```python
from build123d import *

# Parameters (mm, degrees)
SKETCH1_R              = 1.875
SKETCH1_R_2            = 5
BOSS_EXTRUDE1_DEPTH    = 3
CUT_EXTRUDE1_OUTLINE_R = 1.5
CUT_EXTRUDE1_DEPTH     = 3
LPATTERN1_COUNT        = 4
LPATTERN1_PITCH        = 22.666666667
SKETCH1_4_W            = 20
SKETCH1_4_H            = 3
SKETCH1_4_W_2          = 26
BOSS_EXTRUDE2_DEPTH    = 15


# Read off the part's stored shape, not the designer's step: Cut-Extrude1
with BuildPart() as part:
    # Sketch1 → Boss-Extrude1 (new body)
    with BuildSketch(Plane.XY):
        Polygon((77, 130), (63, 130), (63, 127), (37, 127), (37, 130), (23, 130), (23, 127), (3, 127), (3, 130), (0, 130), (0, 0), (100, 0), (100, 130), (97, 130), (97, 127), (77, 127), align=None)
        with Locations((25, 5.75)):
            Circle(SKETCH1_R, mode=Mode.SUBTRACT)
        with Locations((75, 5.75)):
            Circle(SKETCH1_R, mode=Mode.SUBTRACT)
        with BuildLine():
            ThreePointArc((37, 123), (30, 116), (23, 123))
            Line((23, 123), (25, 123))
            ThreePointArc((25, 123), (30, 128), (35, 123))
            Line((35, 123), (37, 123))
        make_face(mode=Mode.SUBTRACT)
        with Locations((70, 123)):
            Circle(SKETCH1_R_2, mode=Mode.SUBTRACT)
    extrude(amount=BOSS_EXTRUDE1_DEPTH)

    # Cut-Extrude1 outline → Cut-Extrude1 (cut)
    with BuildSketch(Plane.XY):
        with Locations((22, 76)):
            Circle(CUT_EXTRUDE1_OUTLINE_R)
        with Locations((10, 92)):
            Circle(CUT_EXTRUDE1_OUTLINE_R)
    cut_extrude1 = extrude(amount=CUT_EXTRUDE1_DEPTH, mode=Mode.SUBTRACT)

    # LPattern1: Cut-Extrude1 ×4
    with Locations(*[(i * LPATTERN1_PITCH, 0, 0) for i in range(1, LPATTERN1_COUNT)]):
        add(cut_extrude1, mode=Mode.SUBTRACT)

    # Sketch1<4> → Boss-Extrude2 (add)
    with BuildSketch(Plane.XY):
        Polygon((0, 130), (0, 90), (3, 90), (3, 127), (3, 130), align=None)
        with Locations((13, 128.5)):
            Rectangle(SKETCH1_4_W, SKETCH1_4_H)
        Polygon((97, 90), (100, 90), (100, 130), (97, 130), (97, 127), align=None)
        with Locations((87, 128.5)):
            Rectangle(SKETCH1_4_W, SKETCH1_4_H)
        with BuildLine():
            Line((77, 127), (77, 130))
            Line((77, 130), (70, 130))
            ThreePointArc((70, 130), (74.949747468, 127.949747468), (77, 123))
            Line((77, 123), (77, 127))
        make_face()
        with BuildLine():
            ThreePointArc((63, 123), (65.050252532, 127.949747468), (70, 130))
            Line((70, 130), (63, 130))
            Line((63, 130), (63, 127))
            Line((63, 127), (63, 123))
        make_face()
        with BuildLine():
            ThreePointArc((77, 123), (74.949747468, 127.949747468), (70, 130))
            ThreePointArc((70, 130), (65.050252532, 127.949747468), (63, 123))
            Line((63, 123), (65, 123))
            ThreePointArc((65, 123), (70, 128), (75, 123))
            Line((75, 123), (77, 123))
        make_face()
        with BuildLine():
            ThreePointArc((63, 123), (70, 116), (77, 123))
            Line((77, 123), (75, 123))
            ThreePointArc((75, 123), (70, 118), (65, 123))
            Line((65, 123), (63, 123))
        make_face()
        with BuildLine():
            ThreePointArc((77, 123), (74.949747468, 127.949747468), (70, 130))
            ThreePointArc((70, 130), (65.050252532, 127.949747468), (63, 123))
            Line((63, 123), (65, 123))
            ThreePointArc((65, 123), (70, 128), (75, 123))
            Line((75, 123), (77, 123))
        make_face()
        with BuildLine():
            ThreePointArc((63, 123), (70, 116), (77, 123))
            Line((77, 123), (75, 123))
            ThreePointArc((75, 123), (70, 118), (65, 123))
            Line((65, 123), (63, 123))
        make_face()
        with Locations((50, 128.5)):
            Rectangle(SKETCH1_4_W_2, SKETCH1_4_H)
        with BuildLine():
            Line((37, 130), (30, 130))
            ThreePointArc((30, 130), (34.949747468, 127.949747468), (37, 123))
            Line((37, 123), (37, 127))
            Line((37, 127), (37, 130))
        make_face()
        with BuildLine():
            Line((30, 130), (23, 130))
            Line((23, 130), (23, 127))
            Line((23, 127), (23, 123))
            ThreePointArc((23, 123), (25.050252532, 127.949747468), (30, 130))
        make_face()
        with BuildLine():
            ThreePointArc((37, 123), (34.949747468, 127.949747468), (30, 130))
            ThreePointArc((30, 130), (25.050252532, 127.949747468), (23, 123))
            Line((23, 123), (25, 123))
            ThreePointArc((25, 123), (30, 128), (35, 123))
            Line((35, 123), (37, 123))
        make_face()
        with BuildLine():
            Line((25, 123), (23, 123))
            ThreePointArc((23, 123), (30, 116), (37, 123))
            Line((37, 123), (35, 123))
            ThreePointArc((35, 123), (30, 118), (25, 123))
        make_face()
        with BuildLine():
            ThreePointArc((37, 123), (34.949747468, 127.949747468), (30, 130))
            ThreePointArc((30, 130), (25.050252532, 127.949747468), (23, 123))
            Line((23, 123), (25, 123))
            ThreePointArc((25, 123), (30, 128), (35, 123))
            Line((35, 123), (37, 123))
        make_face()
        with BuildLine():
            Line((25, 123), (23, 123))
            ThreePointArc((23, 123), (30, 116), (37, 123))
            Line((37, 123), (35, 123))
            ThreePointArc((35, 123), (30, 118), (25, 123))
        make_face()
    extrude(amount=BOSS_EXTRUDE2_DEPTH)


solid = part.part
```
Input: part model. Units: mm. Frame: model coordinates. A direction names the side the tool comes from. Give positions to 0.01 mm unless a question says otherwise; leave off trailing zeros. Order: outer loops, then holes, each group sorted by start corner. A loop starts at its lowest first (then second) coordinate and runs counter-clockwise, first axis right, second up.
1. Section A-A on y = 76. Return the cut outline in (x, z), and give its area (3 significant figures).
Derived:
outline: (0, 0) - (20.5, 0) - (20.5, 3) - (0, 3) - close; (23.5, 0) - (43.17, 0) - (43.17, 3) - (23.5, 3) - close; (46.17, 0) - (65.83, 0) - (65.83, 3) - (46.17, 3) - close; (68.83, 0) - (88.5, 0) - (88.5, 3) - (68.83, 3) - close; (91.5, 0) - (100, 0) - (100, 3) - (91.5, 3) - close
area: 264 mm2
2. Section C-C on z = 9.25. Return the cut outline in (x, y).
Derived:
outline: (0, 90) - (3, 90) - (3, 127) - (23, 127) - (23, 123) arc R7 ccw to (37, 123) - (37, 127) - (63, 127) - (63, 123) arc R7 ccw to (77, 123) - (77, 127) - (97, 127) - (97, 90) - (100, 90) - (100, 130) - (0, 130) - close; hole circle Ø10 at (30, 123); hole circle Ø10 at (70, 123)
3. Pin query (flat end, axial travel): pin 1 (4 mm diameter, centred on x = 22, y = 76, fed in from +Z); pin 2 (2.5 mm diameter, centred on x = 2, z = 10.5, fed in from -Y); pin 3 (1.5 mm diameter, centred on x = 40.5, z = 12, fed in from -Y). Return the tip coordinate at first contact, or that it passes through.
Derived:
pin 1: stops at z = 3
pin 2: stops at y = 90
pin 3: stops at y = 127
4. Section D-D on y = 5.75. Return the cut outline in (x, z) (3 decimals), and give its area (4 significant figures).
Derived:
outline: (0, 0) - (23.125, 0) - (23.125, 3) - (0, 3) - close; (26.875, 0) - (73.125, 0) - (73.125, 3) - (26.875, 3) - close; (76.875, 0) - (100, 0) - (100, 3) - (76.875, 3) - close
area: 277.5 mm2
5. Material intervals for L1, parallel to X at y = 123, z = 7.25; L2, parallel to X at y = 76, z = 0.85; L3, parallel to Y at x = 70, z = 3.5, sorted ascending.
Derived:
L1: x = 0 to 3, 23 to 25, 35 to 37, 63 to 65, 75 to 77, 97 to 100
L2: x = 0 to 20.5, 23.5 to 43.17, 46.17 to 65.83, 68.83 to 88.5, 91.5 to 100
L3: y = 116 to 118, 128 to 130
6. Section B-B on x = 10. Return the cut outline in (y, z), and give its area (3 significant figures).
Derived:
outline: (0, 0) - (90.5, 0) - (90.5, 3) - (0, 3) - close; (93.5, 0) - (130, 0) - (130, 15) - (127, 15) - (127, 3) - (93.5, 3) - close
area: 417 mm2
7. Mould query, pull axis X, two halves, no side actions, for faces 4 (the flat face through (3, 108, 9)), 5 (the flat face through (51, 130, 7)). Classes: released by +X, released by -X, zero draft, split by the parting line, or undercut.
Derived:
face 4: undercut
face 5: zero draft
8. Reachability of faces 1 (the flat face through (1, 90, 9)), 2 (the cylindrical face through (78.806, 93.265, 1.479)), 3 (the flat face through (13, 127, 9)) from +Z, -Z, +X, -X, +Y, -Y: full face, straight path, thin tool, end or side. Return the list, or none.
Derived:
face 1: +Z, +X, -X, -Y
face 2: +Z, -Z
face 3: +Z, -Y
